from build123d import *

# Parameters (mm, degrees)
BOSS_EXTRU_1_DEPTH      = 7
ESQUISSE3_R             = 1.4
ENL_V_MAT_EXTRU_1_DEPTH = 7
ESQUISSE4_R             = 0.95
ENL_V_MAT_EXTRU_2_DEPTH = 7
CONG_1_R                = 3.5
CONG_2_R                = 4
CONG_3_R                = 3


with BuildPart() as part:
    # Esquisse1 → Boss.-Extru.1 (new body)
    with BuildSketch(Plane.XY):
        Polygon((17, 15), (0, 5), (-6, 5), (-6, 0), (0, 0), (17, 10), (27, 10), (27, 15), align=None)
    extrude(amount=BOSS_EXTRU_1_DEPTH)

    # Esquisse3 → Enlèv. mat.-Extru.1 (cut)
    with BuildSketch(Plane(origin=(0, 5, 0), x_dir=(1, 0, 0), z_dir=(0, 1, 0))):
        with Locations(Location((-3, -3, 0), (0, 0, 270))):
            Circle(ESQUISSE3_R)
    extrude(amount=-ENL_V_MAT_EXTRU_1_DEPTH, mode=Mode.SUBTRACT)

    # Esquisse4 → Enlèv. mat.-Extru.2 (cut)
    with BuildSketch(Plane(origin=(0, 15, 0), x_dir=(1, 0, 0), z_dir=(0, 1, 0))):
        with Locations(Location((24, -3.5, 0), (0, 0, 180))):
            Circle(ESQUISSE4_R)
    extrude(amount=-ENL_V_MAT_EXTRU_2_DEPTH, mode=Mode.SUBTRACT)

    # Congé1
    cong_1_edges = [part.edges().sort_by_distance(p)[0] for p in [
        (27, 12.5, 7),
        (27, 12.5, 0),
    ]]
    fillet(cong_1_edges, radius=CONG_1_R - 0.0001)  # a hair under: the kernel refuses the full size

    # Congé2
    cong_2_edges = [part.edges().sort_by_distance(p)[0] for p in [
        (-6, 2.5, 7),
    ]]
    fillet(cong_2_edges, radius=CONG_2_R)

    # Congé3
    cong_3_edges = [part.edges().sort_by_distance(p)[0] for p in [
        (-6, 2.5, 0),
    ]]
    fillet(cong_3_edges, radius=CONG_3_R - 0.0001)  # a hair under: the kernel refuses the full size


solid = part.part
Verification items for the finished model (mm, model axes). A direction names the side the tool comes from. Coordinates: 2 decimals unless noted, no trailing zeros. Write each loop counter-clockwise with the first axis right and the second up, starting at its lowest first coordinate (ties: lowest second). Pieces come first, ordered by that corner, then holes. Notation, with made-up numbers: (31, 46) - (56, 46) arc R7 ccw to (56, 54) - close; hole circle Ø2 at (19.25, -18). An arc over 180 degrees is marked (long way). Answer as a JSON object with one key per item and string values.
(1) Thickness scan on line 1 along Y through (x, z) = (25.5, 2.75); line 2 along Y through (x, z) = (-3.5, 1.25); line 3 along X through (y, z) = (9.5, 3.25). Record the ranges inside material, lowest first.
Report:
{"line 1": "10 to 15", "line 2": "0 to 5", "line 3": "7.65 to 16.15"}
(2) Cross-section at C-C on z = 4. Record the cut outline in (x, y), plus the area to 3 significant figures.
Report:
{"outline": "(-5.87, 0) - (-3.98, 0) - (-3.98, 5) - (-5.87, 5) - close; (-2.02, 0) - (0, 0) - (17, 10) - (23.19, 10) - (23.19, 15) - (17, 15) - (0, 5) - (-2.02, 5) - close; (24.81, 10) - (26.96, 10) - (26.96, 15) - (24.81, 15) - close", "area": "146 mm^2"}
(3) Tool access check on faces 1 (the flat face through (22, 10, 3)), 2 (the flat face through (-1.6, 5, 4.2)), 3 (the cylindrical face through (25.95, 12.54, 6)). Record the directions out of +Z, -Z, +X, -X, +Y, -Y that give a thin tool (end or side, any length) a straight path to the whole face; none if there is none.
Report:
{"face 1": "+Z, -Z, +X, -Y", "face 2": "+Z, -Z, -X, +Y", "face 3": "+Z, +X, +Y, -Y"}
(4) Gauge pin test, flat ends, axial feed: pin 1 Ø3 at (x, z) = (24, 3.5) entering from -Y; pin 2 Ø5 at (x, y) = (11.5, 9.5) entering from -Z; pin 3 Ø1.8 at (x, z) = (-2, 4) entering from +Y; pin 4 Ø3 at (y, z) = (7, 4.5) entering from -X. Record the tip position at first contact, or that the pin passes through.
Report:
{"pin 1": "y = 10", "pin 2": "z = 0", "pin 3": "y = 5", "pin 4": "x = 0.85"}
(5) Cross-section at A-A on x = 24. Record the cut outline in (y, z), plus the area to 3 significant figures.
Report:
{"outline": "(10, 0.04) - (15, 0.04) - (15, 2.55) - (10, 2.55) - close; (10, 4.45) - (15, 4.45) - (15, 6.96) - (10, 6.96) - close", "area": "25.1 mm^2"}
(6) Cross-section at B-B on z = 2. Record the cut outline in (x, y), plus the area to 3 significant figures.
Report:
{"outline": "(-5.83, 0) - (-3.98, 0) - (-3.98, 5) - (-5.83, 5) - close; (-2.02, 0) - (0, 0) - (17, 10) - (26.66, 10) - (26.66, 15) - (17, 15) - (0, 5) - (-2.02, 5) - close", "area": "153 mm^2"}
(7) Mould release check, pull along Z, two halves, no side actions. Record for faces 4 (the flat face through (-1.7, 0, 4.2)), 5 (the cylindrical face through (-4.367, 2.535, 2.697)), 6 (the cylindrical face through (-4.797, 2.465, 5.859)): pulls with the +Z half, pulls with the -Z half, needs draft (parallel to the pull), parting line crosses it, or undercut.
Report:
{"face 4": "needs draft", "face 5": "undercut", "face 6": "pulls with the +Z half"}
